```python
from build123d import *

# Parameters (mm, degrees)
SKETCH1_W           = 35
SKETCH1_H           = 45
BOSS_EXTRUDE1_DEPTH = 7.838444594
SKETCH2_W           = 35
SKETCH2_H           = 11.6848633
BOSS_EXTRUDE2_DEPTH = 40
SKETCH3_R           = 9
CUT_EXTRUDE1_DEPTH  = 2
SKETCH4_R           = 3
SKETCH4_R_2         = 1.7
CUT_EXTRUDE2_DEPTH  = 7.838444594
SKETCH5_R           = 1.7
CUT_EXTRUDE3_DEPTH  = 11.6848633
FILLET1_R           = 1.5


with BuildPart() as part:
    # Sketch1 → Boss-Extrude1 (new body)
    with BuildSketch(Plane(origin=(0, 0, 0), x_dir=(1, 0, 0), z_dir=(0, 1, 0))):
        Rectangle(SKETCH1_W, SKETCH1_H)
    extrude(amount=-BOSS_EXTRUDE1_DEPTH)

    # Sketch2 → Boss-Extrude2 (add)
    with BuildSketch(Plane.XZ.offset(7.838444594)):
        with Locations((0, 16.65756835)):
            Rectangle(SKETCH2_W, SKETCH2_H)
    extrude(amount=BOSS_EXTRUDE2_DEPTH)

    # Sketch3 → Cut-Extrude1 (cut)
    with BuildSketch(Plane.XZ.offset(7.838444594)):
        with Locations(Location((0, -5.84243165, 0), (0, 0, 270))):
            Circle(SKETCH3_R)
    extrude(amount=-CUT_EXTRUDE1_DEPTH, mode=Mode.SUBTRACT)

    # Sketch4 → Cut-Extrude2 (cut)
    with BuildSketch(Plane.XZ.offset(7.838444594)):
        with Locations(Location((0, -5.84243165, 0), (0, 0, 270))):
            Circle(SKETCH4_R)
        with Locations(Location((0, 5.15756835, 0), (0, 0, 270))):
            Circle(SKETCH4_R_2)
        with Locations(Location((11, -5.84243165, 0), (0, 0, 270))):
            Circle(SKETCH4_R_2)
        with Locations(Location((0, -16.84243165, 0), (0, 0, 270))):
            Circle(SKETCH4_R_2)
        with Locations(Location((-11, -5.84243165, 0), (0, 0, 270))):
            Circle(SKETCH4_R_2)
    extrude(amount=-CUT_EXTRUDE2_DEPTH, mode=Mode.SUBTRACT)

    # Sketch5 → Cut-Extrude3 (cut)
    with BuildSketch(Plane(origin=(0, 0, 10.8151367), x_dir=(-1, 0, 0), z_dir=(0, 0, -1))):
        with Locations((-10, -40.338444594)):
            Circle(SKETCH5_R)
        with Locations((10, -40.338444594)):
            Circle(SKETCH5_R)
        with Locations((-10, -15.338444594)):
            Circle(SKETCH5_R)
        with Locations((10, -15.338444594)):
            Circle(SKETCH5_R)
    extrude(amount=-CUT_EXTRUDE3_DEPTH, mode=Mode.SUBTRACT)

    # Fillet1
    fillet1_edges = [part.edges().sort_by_distance(p)[0] for p in [
        (0, -7.838444594, 10.8151367),
    ]]
    fillet(fillet1_edges, radius=FILLET1_R)


solid = part.part
```
The model under review builds one solid part; all positions refer to its coordinate system, in mm. A direction names the side the tool comes from. Round coordinates to 2 decimals unless told otherwise and drop trailing zeros. Order: outer loops, then holes, each group sorted by start corner. A loop starts at its lowest first (then second) coordinate and runs counter-clockwise, first axis right, second up. Notation, with made-up numbers: M 13.5,52 L 42.5,52 A7 cw 42.5,56 Z; hole C -31,30 d2. An arc over 180 degrees is marked long. Use a Markdown table: item, result.
1) Tool access review of faces 4 (the face through (17.5, -13, 15)), 5 (the face through (0, -5.838, -10)), 6 (the face through (-8, -7.838, -10.4)): name each direction out of +Z, -Z, +X, -X, +Y, -Y from which nothing blocks a thin tool from reaching the whole face with its end or side.
Report:
| item | result |
|---|---|
| face 4 | +Z, -Z, +X, +Y, -Y |
| face 5 | -Y |
| face 6 | -Z, +X, -X, -Y |
2) Consider section B-B (z = -16). Write out the cut boundary in (x, y), then the cut area to 3 significant figures.
Report:
| item | result |
|---|---|
| outline | M -17.5,-7.84 L -1.48,-7.84 L -1.48,0 L -17.5,0 Z; M 1.48,-7.84 L 17.5,-7.84 L 17.5,0 L 1.48,0 Z |
| area | 251 mm^2 |
3) Draft analysis for pull direction Y (two halves, no side actions). For faces 1 (the face through (0, -24, 22.5)), 2 (the face through (10.369, -16.998, 16.576)), 3 (the face through (0.2, -8.3, 10.4)), state which applies: released by +Y, released by -Y, zero draft, split by the parting line, or undercut.
Report:
| item | result |
|---|---|
| face 1 | zero draft |
| face 2 | undercut |
| face 3 | released by -Y |
4) Consider section C-C (x = -14). Write out the cut boundary in (y, z).
Report:
| item | result |
|---|---|
| outline | M -47.84,10.82 L -9.34,10.82 A1.5 cw -7.84,9.32 L -7.84,-22.5 L 0,-22.5 L 0,22.5 L -47.84,22.5 Z |
5) Consider section D-D (z = -10.5). Write out the cut boundary in (x, y).
Report:
| item | result |
|---|---|
| outline | M -17.5,-7.84 L -7.7,-7.84 L -7.7,-5.84 L 7.7,-5.84 L 7.7,-7.84 L 17.5,-7.84 L 17.5,0 L -17.5,0 Z |
6) Wall thickness on line 1 along Y through (x, z) = (-10, 14.5); line 2 along Y through (x, z) = (12, -18); line 3 along Z through (x, y) = (-15, -28): over which ranges is each line inside the solid? List them lowest first. Write a range as [from, to].
Report:
| item | result |
|---|---|
| line 1 | [-47.84, -42.04], [-38.64, -17.04], [-13.64, 0] |
| line 2 | [-7.84, 0] |
| line 3 | [10.82, 22.5] |
7) Insertion check: pin 1 (4.5 mm diameter, centred on x = -10, y = -40.34, fed in from -Z); pin 2 (14.5 mm diameter, centred on x = -4, z = -10, fed in from -Y); pin 3 (11 mm diameter, centred on x = 0, z = -5.84, fed in from -Y). Each pin has a flat end and moves straight along its axis. Give the tip position at first contact, or say it passes through.
Report:
| item | result |
|---|---|
| pin 1 | z = 10.82 |
| pin 2 | y = -7.84 |
| pin 3 | y = -5.84 |
8) Consider section A-A (x = 0). Write out the cut boundary in (y, z).
Report:
| item | result |
|---|---|
| outline | M -47.84,10.82 L -9.34,10.82 A1.5 cw -7.84,9.32 L -7.84,6.86 L 0,6.86 L 0,22.5 L -47.84,22.5 Z; M -7.84,-22.5 L 0,-22.5 L 0,-18.54 L -7.84,-18.54 Z; M -7.84,-15.14 L 0,-15.14 L 0,-8.84 L -5.84,-8.84 L -5.84,-14.84 L -7.84,-14.84 Z; M -7.84,3.16 L -5.84,3.16 L -5.84,-2.84 L 0,-2.84 L 0,3.46 L -7.84,3.46 Z |
